Geometry check sheet. Reference: the model listing, model coordinates, mm. Round coordinates to 2 decimals unless told otherwise and drop trailing zeros. Order: outer loops, then holes, each group sorted by start corner. A loop starts at its lowest first (then second) coordinate and runs counter-clockwise, first axis right, second up.
(1) Gauge pin test, flat ends, axial feed: P1, Ø6, axis at x = 590, z = -127.5, coming from the +Y side; P2, Ø10, axis at y = 612, z = -89, coming from the +X side; P3, Ø2, axis at y = 597.5, z = -115.5, coming from the -X side. Record the tip position at first contact, or that the pin passes through.
(2) Cross-section at C-C on z = -21. Enter the section's corners in (x, y).
(3) Cross-section at B-B on x = 565. Enter the section's corners in (y, z).
(4) Cross-section at D-D on x = 651. Enter the section's corners in (y, z).
(5) Thickness scan on L1, parallel to Y at x = 673, z = -77; L2, parallel to X at y = 606.5, z = -120; L3, parallel to Y at x = 528.5, z = -34.5. Record the ranges inside material, lowest first.
(6) Cross-section at A-A on z = -124. Enter the section's corners in (x, y).
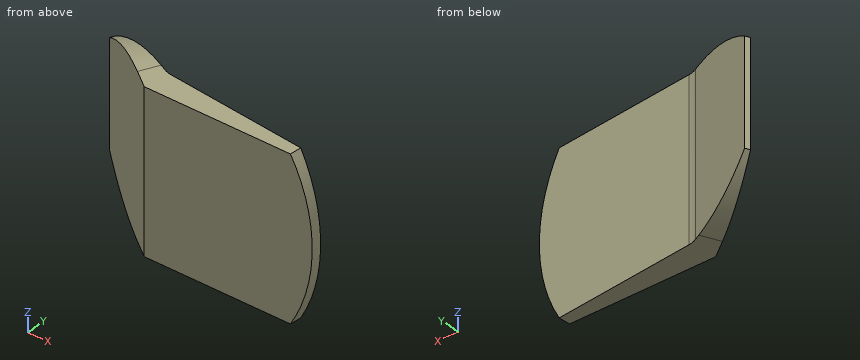
from build123d import *

# Parameters (mm, degrees)
EXTRUDE1_DEPTH = 177.8
EXTRUDE5_DEPTH = 44.45
EXTRUDE6_DEPTH = 44.45


with BuildPart() as part:
    # Sketch1 → Extrude1 (new body)
    with BuildSketch(Plane.XY):
        with BuildLine():
            Line((433.551122257, 624.054848578), (524.118132596, 578.074674098))
            ThreePointArc((524.118132596, 578.074674098), (528.478538405, 576.346602597), (533.082342852, 575.449744447))
            Line((533.082342852, 575.449744447), (710.83449651, 557.626357766))
            Line((710.83449651, 557.626357766), (710.83449651, 547.410087665))
            Line((710.83449651, 547.410087665), (526.236430387, 547.410087665))
            Line((526.236430387, 547.410087665), (431.053198967, 619.134696642))
            Line((431.053198967, 619.134696642), (433.551122257, 624.054848578))
        make_face()
    extrude(amount=-EXTRUDE1_DEPTH)

    # Sketch5 → Extrude5 (cut)
    with BuildSketch(Plane(origin=(62.432960723, 622.642229918, 0), x_dir=(-0.9950104563205879, 0.09977069616222714, 0), z_dir=(0.09977069616222714, 0.9950104563205879, 0))):
        with BuildLine():
            Line((-627.873539531, 0), (-668.145359753, 0))
            Line((-668.145359753, 0), (-668.145359753, -177.8))
            Line((-668.145359753, -177.8), (-627.873539531, -177.8))
            ThreePointArc((-627.873539531, -177.8), (-651.57623812, -88.9), (-627.873539531, 0))
        make_face()
    extrude(amount=-EXTRUDE5_DEPTH, mode=Mode.SUBTRACT)

    # Sketch7 → Extrude6 (cut)
    with BuildSketch(Plane(origin=(340.747990654, 671.170284622, 0), x_dir=(-0.8916667692581813, 0.45269235977723044, 0), z_dir=(0.45269235977723044, 0.8916667692581813, 0))):
        with BuildLine():
            Line((-104.078266458, -30.241656288), (-104.078266458, 0))
            Line((-104.078266458, 0), (-198.470653172, 0))
            ThreePointArc((-198.470653172, 0), (-149.071209803, -8.243889089), (-104.078266458, -30.241656288))
        make_face()
        with BuildLine():
            Line((-104.078266458, -177.8), (-104.078266458, -147.558343712))
            ThreePointArc((-104.078266458, -147.558343712), (-149.071209803, -169.556110911), (-198.470653172, -177.8))
            Line((-198.470653172, -177.8), (-104.078266458, -177.8))
        make_face()
    extrude(amount=-EXTRUDE6_DEPTH, mode=Mode.SUBTRACT)


solid = part.part
Found:
1. P1: stops at y = 570.04
1. P2: stops at x = 467.14
1. P3: stops at x = 458.44
2. outline: (443.33, 609.89) - (526.24, 547.41) - (696.25, 547.41) - (697.41, 558.97) - (533.08, 575.45) arc R25.4 cw to (524.12, 578.07) - (447.04, 617.21) - close
3. outline: (547.41, -177.8) - (572.25, -177.8) - (572.25, 0) - (547.41, 0) - close
4. outline: (547.41, -177.8) - (563.63, -177.8) - (563.63, 0) - (547.41, 0) - close
5. L1: y = 547.41 to 561.42
5. L2: x = 447.82 to 468.13
5. L3: y = 547.41 to 576.34
6. outline: (431.05, 619.13) - (526.24, 547.41) - (706.23, 547.41) - (707.29, 557.98) - (533.08, 575.45) arc R25.4 cw to (524.12, 578.07) - (433.55, 624.05) - close
